Autodesk Inventor part; units mm, degrees
ref_plane "YZ Plane" through (0, 0, 0) normal (1, 0, 0) x (0, 1, 0)
ref_plane "XY Plane" through (0, 0, 0) normal (0, 0, 1) x (1, 0, 0)
sketch "Sketch1" plane through (0, 0, 0) normal (0, 1, 0) x (-1, 0, 0)
  point P0 (0, 0)
sketch "Sketch2" plane through (0, 0, 0) normal (0, 1, 0) x (-1, 0, 0)
  line L0 (-16.4647, 13.2032) -> (-10.9085, 13.2032)
  line L1 (-10.9085, 7.647) -> (-10.9085, -12.1968)
  line L2 (-10.9085, -12.1968) -> (-16.4647, -12.1968)
  line L3 (-16.4647, -12.1968) -> (-16.4647, 13.2032)
  line L4 (-16.4647, 13.2032) -> (8.9353, 13.2032)
  line L5 (8.9353, 13.2032) -> (8.9353, 7.647)
  line L6 (8.9353, 7.647) -> (-10.9085, 7.647)
  line L7 (-16.4647, 7.647) -> (-16.4647, 13.2032)
  point P0 (0, 0)
  dimension "d0" = 5.5563
  dimension "d1" = 25.4
  dimension "d3" = 25.4
  dimension "d4" = 5.5563
extrude "Extrusion1" add sketch "Sketch2" along normal mid plane 25.4
sketch "Sketch3" plane through (16.4647, -12.7, 13.2032) normal (1, 0, 0) x (0, 0, -1)
  line L0 (25.4, 0) -> (0, 0)
  line L1 (25.4, 0) -> (25.4, 25.4)
  point P0 (13.2032, 12.7)
  point P1 (12.7, 12.7)
  point P2 (0, 0)
  dimension "d7" = 12.7
  dimension "d8" = 12.7
sketch "Sketch4" plane through (-8.9353, -12.7, 13.2032) normal (0, 0, 1) x (1, 0, 0)
  line L0 (25.4, 25.4) -> (25.4, 0)
  line L1 (25.4, 0) -> (0, 0)
  point P0 (8.9353, 12.7)
  point P1 (12.7, 12.7)
  dimension "d9" = 12.7
  dimension "d10" = 12.7
hole "Hole1" at (3.7647, 0, 13.2032) direction (0, 0, -1) diameter 6.35 end through all
hole "Hole2" at (16.4647, 0, 0.5032) direction (-1, 0, 0) diameter 6.35 end through all
fillet "Fillet1" radius 4.7625 2 edges at (10.9085, 0, -12.1968) (-8.9353, 0, 7.647)
sketch "Sketch5" plane through (16.4647, -12.7, 13.2032) normal (1, 0, 0) x (0, 0, -1)
  line L0 (20.6375, 25.4) -> (5.5562, 25.4)
  line L1 (9.652, 25.4) -> (9.652, 0)
  line L2 (5.5562, 0) -> (20.6375, 0)
  line L3 (15.748, 25.4) -> (15.748, 0)
  line L4 (0, 25.4) -> (0, 0)
  line L5 (9.652, 25.4) -> (15.748, 25.4)
  line L6 (15.748, 0) -> (9.652, 0)
  point P0 (13.2032, 12.7)
  dimension "d26" = 6.096
  dimension "d27" = 9.652
extrude "Extrusion2" add sketch "Sketch5" along normal blind 3.175
properties part number "rope connection to cart"
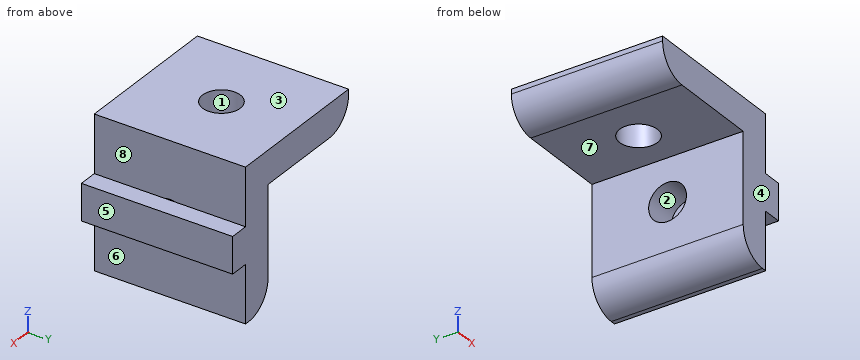
Work out the finished part from the listing and answer in its coordinate system (mm). Face numbers are marked on the shaded views. A direction names the side the tool comes from. Give positions to 0.01 mm unless a question says otherwise; leave off trailing zeros. Write each loop counter-clockwise with the first axis right and the second up, starting at its lowest first coordinate (ties: lowest second). Pieces come first, ordered by that corner, then holes. Notation, with made-up numbers: M 61.25,11 L 71.25,11 A25 ccw 71.25,31 Z; hole C -39,-36.5 d3. An arc over 180 degrees is marked long. Answer as CSV lines item,"result".
Q1. The mould has two halves that part along Z. Classify the marked faces 1, 2 and 3: +Z half, -Z half, draft (parallel to the pull), parting line (faces both ways), or undercut.
A:
face 1,"draft"
face 2,"undercut"
face 3,"+Z half"
Q2. A cutting plane is placed at B-B on x = 2.5. Write down the section's boundary in (y, z).
A:
outline,"M -12.7,7.65 L -2.91,7.65 L -2.91,13.2 L -12.7,13.2 Z; M 2.91,7.65 L 12.7,7.65 L 12.7,13.2 L 2.91,13.2 Z"
Q3. Given P1, Ø7.5, axis at y = 1, z = 8, coming from the +X side; P2, Ø1, axis at y = 7.5, z = -3, coming from the -X side; P3, Ø1.5, axis at x = 4, y = 9.5, coming from the -Z side; P4, Ø6, axis at x = 13, y = 8.5, coming from the -Z side, each flat-ended and moving along its own axis, determine where each tip first touches the part or whether it passes through.
A:
P1,"stops at x = 16.46"
P2,"stops at x = 10.91"
P3,"stops at z = 7.65"
P4,"stops at z = -12.2"
Q4. A tool of negligible diameter and unlimited length cuts with its end or side. For the marked faces 4, 5, 6, 7 and 8, from which of +Z, -Z, +X, -X, +Y, -Y can it reach the whole face along a straight path? Write none if from no direction.
A:
face 4,"+Z, -Z, +X, -X, -Y"
face 5,"+Z, -Z, +X, +Y, -Y"
face 6,"-Z, +X, +Y, -Y"
face 7,"-Z, -X, +Y, -Y"
face 8,"+Z, +X, +Y, -Y"
Q5. A cutting plane is placed at D-D on y = 2.75. Write down the section's boundary in (x, z) (1 decimal).
A:
outline,"M -8.9,12.4 A4.8 ccw -4.2,7.6 L 2.2,7.6 L 2.2,13.2 L -8.9,13.2 Z; M 5.4,7.6 L 10.9,7.6 L 10.9,2.1 L 16.5,2.1 L 16.5,-1.1 L 10.9,-1.1 L 10.9,-7.4 A4.8 ccw 15.7,-12.2 L 16.5,-12.2 L 16.5,-2.5 L 19.6,-2.5 L 19.6,3.6 L 16.5,3.6 L 16.5,13.2 L 5.4,13.2 Z"
Q6. A cutting plane is placed at A-A on y = 0. Write down the section's boundary in (x, z) (1 decimal), plus the area to 3 significant figures.
A:
outline,"M -8.9,12.4 A4.8 ccw -4.2,7.6 L 0.6,7.6 L 0.6,13.2 L -8.9,13.2 Z; M 6.9,7.6 L 10.9,7.6 L 10.9,3.7 L 16.5,3.7 L 16.5,13.2 L 6.9,13.2 Z; M 10.9,-7.4 A4.8 ccw 15.7,-12.2 L 16.5,-12.2 L 16.5,-2.7 L 10.9,-2.7 Z; M 16.5,-2.5 L 19.6,-2.5 L 19.6,3.6 L 16.5,3.6 Z"
area,"190 mm²"
Q7. A cutting plane is placed at C-C on y = 7.25. Write down the section's boundary in (x, z) (1 decimal).
A:
outline,"M -8.9,12.4 A4.8 ccw -4.2,7.6 L 10.9,7.6 L 10.9,-7.4 A4.8 ccw 15.7,-12.2 L 16.5,-12.2 L 16.5,-2.5 L 19.6,-2.5 L 19.6,3.6 L 16.5,3.6 L 16.5,13.2 L -8.9,13.2 Z"
Q8. Find the intervals of material crossed by probe 1 along X at (y, z) = (-9, 3.25); probe 2 along X at (y, z) = (-6.5, 5); probe 3 along Z at (x, y) = (10.75, 10), in increasing order. Write a range as [from, to].
A:
probe 1,"x = [10.91, 19.64]"
probe 2,"x = [10.91, 16.46]"
probe 3,"z = [7.65, 13.2]"
